Can you work these out from the model? Positions are in its coordinate system, mm. Face numbers are marked on the shaded views. A direction names the side the tool comes from. Give positions to 0.01 mm unless a question says otherwise; leave off trailing zeros. Loops run counter-clockwise (first coordinate to the right, second up) from the corner with the lowest first, then second, coordinate; pieces in that order, holes last. Notation, with made-up numbers: (86.25, -20.75) - (112.25, -20.75) arc R28 cw to (112.25, 11.25) - close; hole circle Ø3 at (-40, 88.5). An arc over 180 degrees is marked (long way). Answer as a JSON object with one key per item and string values. Group by question number.
Item 1: Suppose I cut it at C-C on y = 9.5. Write out the boundary of the cut face in (x, z).
Item 2: Thinking about a two-plate mould opening in Z: for the marked faces 1, 2 and 3, which applies, pulls with the +Z half, pulls with the -Z half, needs draft (parallel to the pull), parting line crosses it, or undercut?
Item 3: Suppose I cut it at A-A on x = -0.5. Write out the boundary of the cut face in (y, z), and give its area (3 significant figures).
Item 4: Suppose I cut it at D-D on x = -8.5. Write out the boundary of the cut face in (y, z).
Item 5: Suppose I cut it at B-B on z = -0.5. Write out the boundary of the cut face in (x, y).
Item 6: Will these pins go through, and if not, where does the flat tip stop? pin 1 (3 mm diameter, centred on x = -4.5, z = -9.5, fed in from -Y); pin 2 (2.5 mm diameter, centred on x = 1, y = 18, fed in from -Z); pin 3 (4 mm diameter, centred on y = -2, z = 4, fed in from -X).
Item 7: Please list where these lines run through material, in increasing order: L1, parallel to X at y = 25, z = -0.5; L2, parallel to Y at x = 5.5, z = -3; L3, parallel to X at y = -3.5, z = 6.
Item 8: Which directions (+Z, -Z, +X, -X, +Y, -Y) give clear straight access to the entire face, cutting with the end or side of a thin tool? Please do the marked faces 4, 5, 6, 7 and 8.
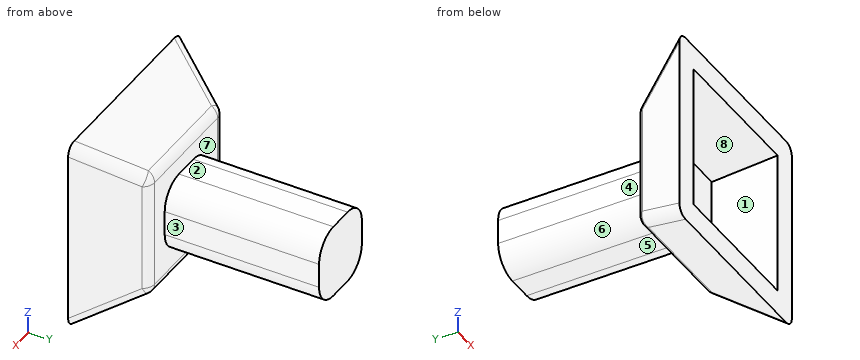
from build123d import *

# Parameters (mm, degrees)
SKETCH1_W           = 15.24
SKETCH1_H           = 15.24
BOSS_EXTRUDE1_DEPTH = 31.75
FILLET1_R           = 5.08
SKETCH2_W           = 25.4
SKETCH2_H           = 25.4
BOSS_EXTRUDE3_DEPTH = 12.7
BOSS_EXTRUDE3_DRAFT = -30
SKETCH5_W           = 29.904696838
SKETCH5_H           = 29.904696838
CUT_EXTRUDE1_DEPTH  = 10.16
CUT_EXTRUDE1_DRAFT  = -30
FILLET2_R           = 2.54


with BuildPart() as part:
    # Sketch1 → Boss-Extrude1 (new body)
    with BuildSketch(Plane(origin=(0, 0, 0), x_dir=(1, 0, 0), z_dir=(0, 1, 0))):
        Rectangle(SKETCH1_W, SKETCH1_H)
    extrude(amount=BOSS_EXTRUDE1_DEPTH)

    # Fillet1
    fillet1_edges = [part.edges().sort_by_distance(p)[0] for p in [
        (-7.62, 15.875, -7.62),
        (7.62, 15.875, -7.62),
        (7.62, 15.875, 7.62),
        (-7.62, 15.875, 7.62),
    ]]
    fillet(fillet1_edges, radius=FILLET1_R)


with BuildPart() as boss_extrude3_tool:
    # Sketch2 → Boss-Extrude3 (with draft: the straight prism first)
    with BuildSketch(Plane.XZ):
        Rectangle(SKETCH2_W, SKETCH2_H)
    extrude(amount=BOSS_EXTRUDE3_DEPTH)
    # Boss-Extrude3: the draft: its side faces are tilted about the plane it starts from
    boss_extrude3_sides = [boss_extrude3_tool.faces().sort_by_distance(p)[0] for p in [
        (12.7, -6.35, 0),
        (0, -6.35, 12.7),
        (-12.7, -6.35, 0),
        (0, -6.35, -12.7),
    ]]
    draft(boss_extrude3_sides, Plane.XZ, BOSS_EXTRUDE3_DRAFT)


with BuildPart() as part_1:
    add(part.part)

    # Boss-Extrude3: add boss_extrude3_tool
    add(boss_extrude3_tool.part)


with BuildPart() as cut_extrude1_tool:
    # Sketch5 → Cut-Extrude1 (with draft: the straight prism first)
    with BuildSketch(Plane.XZ.offset(12.7)):
        Rectangle(SKETCH5_W, SKETCH5_H)
    extrude(amount=-CUT_EXTRUDE1_DEPTH)
    # Cut-Extrude1: the draft: its side faces are tilted about the plane it starts from
    cut_extrude1_sides = [cut_extrude1_tool.faces().sort_by_distance(p)[0] for p in [
        (-14.952348419, -7.62, 0),
        (0, -7.62, -14.952348419),
        (14.952348419, -7.62, 0),
        (0, -7.62, 14.952348419),
    ]]
    draft(cut_extrude1_sides, Plane.XZ.offset(12.7), CUT_EXTRUDE1_DRAFT)


with BuildPart() as part_2:
    add(part_1.part)

    # Cut-Extrude1: cut by cut_extrude1_tool
    add(cut_extrude1_tool.part, mode=Mode.SUBTRACT)

    # Fillet2
    fillet2_edges = [part_2.edges().sort_by_distance(p)[0] for p in [
        (-12.7, 0, 0),
        (-16.366174209, -6.35, 16.366174209),
        (0, 0, -12.7),
        (-16.366174209, -6.35, -16.366174209),
        (12.7, 0, 0),
        (16.366174209, -6.35, -16.366174209),
        (0, 0, 12.7),
        (16.366174209, -6.35, 16.366174209),
    ]]
    fillet(fillet2_edges, radius=FILLET2_R)


solid = part_2.part
Worked out:
{
 "1": {"outline": "(-7.62, -2.54) arc R5.08 ccw to (-2.54, -7.62) - (2.54, -7.62) arc R5.08 ccw to (7.62, -2.54) - (7.62, 2.54) arc R5.08 ccw to (2.54, 7.62) - (-2.54, 7.62) arc R5.08 ccw to (-7.62, 2.54) - close"},
 "2": {"face 1": "undercut", "face 2": "pulls with the +Z half", "face 3": "needs draft"},
 "3": {"outline": "(-12.7, -20.03) - (-1.27, -13.43) arc R2.54 ccw to (0, -11.23) - (0, -7.62) - (31.75, -7.62) - (31.75, 7.62) - (0, 7.62) - (0, 11.23) arc R2.54 ccw to (-1.27, 13.43) - (-12.7, 20.03) - (-12.7, 14.95) - (-2.54, 9.09) - (-2.54, -9.09) - (-12.7, -14.95) - close", "area": "655 mm2"},
 "4": {"outline": "(-12.7, -20.03) - (-1.27, -13.43) arc R2.54 ccw to (0, -11.23) - (0, 11.23) arc R2.54 ccw to (-1.27, 13.43) - (-12.7, 20.03) - (-12.7, 14.95) - (-2.54, 9.09) - (-2.54, -9.09) - (-12.7, -14.95) - close"},
 "5": {"outline": "(-20.03, -12.7) - (-14.95, -12.7) - (-9.09, -2.54) - (9.09, -2.54) - (14.95, -12.7) - (20.03, -12.7) - (13.43, -1.27) arc R2.54 ccw to (11.23, 0) - (7.62, 0) - (7.62, 31.75) - (-7.62, 31.75) - (-7.62, 0) - (-11.23, 0) arc R2.54 ccw to (-13.43, -1.27) - close"},
 "6": {"pin 1": "stops at y = -5.85", "pin 2": "stops at z = -7.62", "pin 3": "stops at x = -15.01"},
 "7": {"L1": "x = -7.62 to 7.62", "L2": "y = -2.54 to 31.75", "L3": "x = -14.72 to -9.64, 9.64 to 14.72"},
 "8": {"face 4": "+Z, -Z, -X, +Y", "face 5": "-Z, +X, -X, +Y", "face 6": "-Z, -X, +Y", "face 7": "+Y", "face 8": "-Y"}
}
